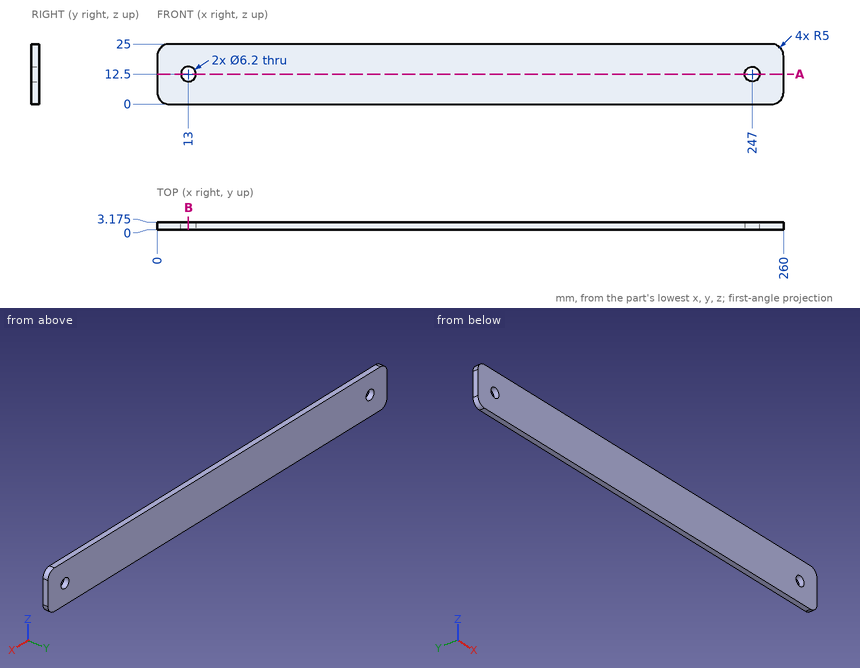
Geometry: see drawing. Coordinates: mm, zero at the bounding-box minimum. Give positions to 0.01 mm unless a question says otherwise; leave off trailing zeros. Write each loop counter-clockwise with the first axis right and the second up, starting at its lowest first coordinate (ties: lowest second). Pieces come first, ordered by that corner, then holes. Notation, with made-up numbers: (-29.5, 83.5) -> (-23.5, 83.5) arc R24 ccw to (-23.5, 111.5) -> close; hole circle Ø10 at (-26.5, 27.5). An arc over 180 degrees is marked (long way). Use one line per item in the form item = value. Start each with the question number.
1) Section query B-B on x = 13. Return the cut outline in (y, z) (3 decimals), then the cut area to 3 significant figures.
2) Section query A-A on z = 12.5. Return the cut outline in (x, y) (3 decimals).
3) Ray query, probe 1 along Z at (x, y) = (13, 1.95); probe 2 along X at (y, z) = (1.95, 4.5); probe 3 along Z at (x, y) = (245.5, 2.6). Return the intervals inside material, ascending. Write a range as from..to.
Outcome:
q1.outline = (0, 0) -> (3.175, 0) -> (3.175, 9.4) -> (0, 9.4) -> close; (0, 15.6) -> (3.175, 15.6) -> (3.175, 25) -> (0, 25) -> close
q1.area = 59.7 mm^2
q2.outline = (0, 0) -> (9.9, 0) -> (9.9, 3.175) -> (0, 3.175) -> close; (16.1, 0) -> (243.9, 0) -> (243.9, 3.175) -> (16.1, 3.175) -> close; (250.1, 0) -> (260, 0) -> (260, 3.175) -> (250.1, 3.175) -> close
q3.probe_1 = 0..9.4, 15.6..25
q3.probe_2 = 0.03..259.97
q3.probe_3 = 0..9.79, 15.21..25
